```python
from build123d import *
from OCP.BRepFilletAPI import BRepFilletAPI_MakeChamfer

# Parameters (mm, degrees)
BOSS_EXTRUDE1_DEPTH     = 16.399996177
CUT_EXTRUDE1_DEPTH      = 32.345970628
CUT_EXTRUDE3_DEPTH      = 30.26106414
CUT_EXTRUDE3_DEPTH_BACK = 30.26106414
SKETCH4_R               = 1.7
BOSS_EXTRUDE2_START     = -4
BOSS_EXTRUDE2_DEPTH     = 4
FILLET1_R               = 12
CHAMFER1_SIZE           = 0.5
CHAMFER2_SIZE           = 0.5
CHAMFER2_SIZE2          = 1.366025404
MIRROR2_START           = 1.4
MIRROR2_DEPTH           = 9
CUT_EXTRUDE4_DEPTH      = 31.847364144
BOSS_EXTRUDE4_DEPTH     = 2.3
CHAMFER3_SIZE           = 2.3


# Read off the part's stored shape, not the designer's step: Mirror2
with BuildPart() as part:
    # Sketch1 → Boss-Extrude1 (new body)
    with BuildSketch(Plane.XY.offset(16.399996177)):
        with BuildLine():
            Line((7.2, 1.4), (22.5, 1.4))
            Line((22.5, 1.4), (22.5, 14.4))
            Line((22.5, 14.4), (7.2, 14.4))
            ThreePointArc((7.2, 14.4), (0.7, 7.9), (7.2, 1.4))
        make_face()
    extrude(amount=-BOSS_EXTRUDE1_DEPTH)

    # Sketch2 → Cut-Extrude1 (cut, through all)
    with BuildSketch(Plane(origin=(0, 0, 0), x_dir=(-1, 0, 0), z_dir=(0, 0, -1))):
        with BuildLine():
            Line((-22.5, 10.4), (-22.5, 5.4))
            Line((-22.5, 5.4), (-10.532688106, 5.4))
            ThreePointArc((-10.532688106, 5.4), (-2.9577807, 7.9), (-10.532688106, 10.4))
            Line((-10.532688106, 10.4), (-22.5, 10.4))
        make_face()
    extrude(amount=-CUT_EXTRUDE1_DEPTH, mode=Mode.SUBTRACT)

    # Sketch4 → Cut-Extrude3 (cut, two sides: drawn at the far end of the back side and taken through both)
    with BuildSketch(Plane.XZ.offset(-10.4).offset(-CUT_EXTRUDE3_DEPTH_BACK)):
        with Locations((19.72, 8.2)):
            Circle(SKETCH4_R)
    extrude(amount=CUT_EXTRUDE3_DEPTH + CUT_EXTRUDE3_DEPTH_BACK, mode=Mode.SUBTRACT)

    # Sketch5 → Boss-Extrude2 (add)
    with BuildSketch(Plane(origin=(0, 14.4, 0), x_dir=(1, 0, 0), z_dir=(0, 1, 0)).offset(BOSS_EXTRUDE2_START)):
        Polygon((22.5, 0), (22.5, -16.399996177), (27.234271104, -8.199998088), align=None)
    extrude(amount=BOSS_EXTRUDE2_DEPTH)

    # Fillet1
    fillet1_edges = [part.edges().sort_by_distance(p)[0] for p in [
        (27.234271104, 12.4, 8.199998088),
    ]]
    fillet(fillet1_edges, radius=FILLET1_R)

    # Chamfer1
    chamfer1_edges = [part.edges().sort_by_distance(p)[0] for p in [
        (2.9577807, 7.9, 16.399996177),
    ]]
    chamfer(chamfer1_edges, length=CHAMFER1_SIZE)

    # Chamfer2: one chamfer whose edges measure the first distance from different faces: ONE call of the kernel's chamfer builder (chamfer() names one face for all edges)
    chamfer2_edges_1 = [part.edges().sort_by_distance(p)[0] for p in [
        (22.5, 12.4, 16.399996177),
    ]]
    chamfer2_side_1 = [part.faces().sort_by_distance(p)[0] for p in [
        (23.135084744, 12.4, 15.299997133),
    ]]
    chamfer2_edges_2 = [part.edges().sort_by_distance(p)[0] for p in [
        (14.85, 1.4, 16.399996177),
        (0.7, 7.9, 16.399996177),
        (14.85, 14.4, 16.399996177),
        (16.818865224, 10.4, 16.399996177),
        (16.818865224, 5.4, 16.399996177),
    ]]
    chamfer2 = BRepFilletAPI_MakeChamfer(part.part.solid().wrapped)
    for e in chamfer2_edges_1:
        chamfer2.Add(CHAMFER2_SIZE, CHAMFER2_SIZE2, e.wrapped, chamfer2_side_1[0].wrapped)  # the first distance lies on this face
    for e in chamfer2_edges_2:
        chamfer2.Add(CHAMFER2_SIZE, e.wrapped)
    add(Compound.cast(chamfer2.Shape()), mode=Mode.REPLACE)

    # Mirror2 outline → Mirror2 (add)
    with BuildSketch(Plane(origin=(0, 0, 0), x_dir=(1, 0, 0), z_dir=(0, 1, 0)).offset(MIRROR2_START)):
        with BuildLine():
            ThreePointArc((23.770169489, -14.199998088), (25.377864643, -8.199998088), (23.770169489, -2.199998088))
            Line((23.770169489, -2.199998088), (22.5, 0))
            Line((22.5, 0), (22.5, -16.399996177))
            Line((22.5, -16.399996177), (23.770169489, -14.199998088))
        make_face()
    extrude(amount=MIRROR2_DEPTH)

    # Sketch7 → Cut-Extrude4 (cut, through all)
    with BuildSketch(Plane.ZY.offset(-22.5)):
        Polygon((0, 10.4), (0, 5.4), (15.899996177, 5.4), (16.399996177, 4.9), (16.399996177, 10.4), (15.899996177, 10.4), align=None)
    extrude(amount=-CUT_EXTRUDE4_DEPTH, mode=Mode.SUBTRACT)

    # Sketch9 → Boss-Extrude4 (add)
    with BuildSketch(Plane.XZ.offset(-1.4)):
        Polygon((16.891066023, 3.300146444), (22.548930666, 3.300144532), (25.377864643, 8.199998088), (22.548933977, 13.099853556), (16.891069334, 13.099855468), (14.062135357, 8.200001912), align=None)
        Polygon((21.32, 10.971281292), (18.12, 10.971281292), (16.52, 8.2), (18.12, 5.428718708), (21.32, 5.428718708), (22.92, 8.2), align=None, mode=Mode.SUBTRACT)
    extrude(amount=BOSS_EXTRUDE4_DEPTH)

    # Chamfer3
    # the kernel refuses this chamfer: 2.3 mm, written as the material it takes off along each edge
    with BuildSketch(Plane(origin=(19.591493499, -0.9, -1.822282904), x_dir=(0.023812122999065932, 0.9996219169112968, -0.013747946350707228), z_dir=(0.5000002926043912, 0, 0.8660252348491488))) as chamfer3_piece_1_section:
        Polygon((CHAMFER3_SIZE * 0.999621916911, CHAMFER3_SIZE * 0.0274958766106), (-CHAMFER3_SIZE * 0.0274958766106, CHAMFER3_SIZE * 0.999621916911), (0, 0), align=None)
    chamfer3_piece_1 = extrude(amount=17.487606388, mode=Mode.PRIVATE)
    chamfer3_piece_1 = split(chamfer3_piece_1, bisect_by=Plane(origin=(23.305279483, 1.4, 6.13003631), z_dir=(0, -1, 0)), keep=Keep.TOP, mode=Mode.PRIVATE)
    add(chamfer3_piece_1, mode=Mode.SUBTRACT)
    with BuildSketch(Plane(origin=(10.976195151, -0.9, 3.300148442), x_dir=(-9.290045060267903e-09, 0.9996219169112968, -0.027495876610584728), z_dir=(0.999999999999943, 0, -3.378704806423189e-07))) as chamfer3_piece_2_section:
        Polygon((CHAMFER3_SIZE * 0.999621916911, CHAMFER3_SIZE * 0.0274958766106), (-CHAMFER3_SIZE * 0.0274958766106, CHAMFER3_SIZE * 0.999621916911), (0, 0), align=None)
    chamfer3_piece_2 = extrude(amount=17.487606388, mode=Mode.PRIVATE)
    chamfer3_piece_2 = split(chamfer3_piece_2, bisect_by=Plane(origin=(19.719998601, 1.4, 4.060075043), z_dir=(0, -1, 0)), keep=Keep.TOP, mode=Mode.PRIVATE)
    add(chamfer3_piece_2, mode=Mode.SUBTRACT)
    with BuildSketch(Plane(origin=(11.104701651, -0.9, 13.322431346), x_dir=(-0.023812132289111273, 0.9996219169112968, -0.013747930259877354), z_dir=(0.49999970739555216, 0, -0.8660255727196295))) as chamfer3_piece_3_section:
        Polygon((CHAMFER3_SIZE * 0.999621916911, CHAMFER3_SIZE * 0.0274958766106), (-CHAMFER3_SIZE * 0.0274958766106, CHAMFER3_SIZE * 0.999621916911), (0, 0), align=None)
    chamfer3_piece_3 = extrude(amount=17.487606388, mode=Mode.PRIVATE)
    chamfer3_piece_3 = split(chamfer3_piece_3, bisect_by=Plane(origin=(16.134719118, 1.4, 6.130038733), z_dir=(0, -1, 0)), keep=Keep.TOP, mode=Mode.PRIVATE)
    add(chamfer3_piece_3, mode=Mode.SUBTRACT)
    with BuildSketch(Plane(origin=(19.848506501, -0.9, 18.222282904), x_dir=(-0.023812122999067282, 0.9996219169112966, 0.013747946350707963), z_dir=(-0.5000002926043904, 0, -0.8660252348491492))) as chamfer3_piece_4_section:
        Polygon((CHAMFER3_SIZE * 0.999621916911, CHAMFER3_SIZE * 0.0274958766106), (-CHAMFER3_SIZE * 0.0274958766106, CHAMFER3_SIZE * 0.999621916911), (0, 0), align=None)
    chamfer3_piece_4 = extrude(amount=17.487606388, mode=Mode.PRIVATE)
    chamfer3_piece_4 = split(chamfer3_piece_4, bisect_by=Plane(origin=(16.134720517, 1.4, 10.26996369), z_dir=(0, -1, 0)), keep=Keep.TOP, mode=Mode.PRIVATE)
    add(chamfer3_piece_4, mode=Mode.SUBTRACT)
    with BuildSketch(Plane(origin=(28.335298349, -0.9, 3.077568654), x_dir=(0.02381213228911159, 0.9996219169112966, 0.013747930259877545), z_dir=(-0.499999707395552, 0, 0.8660255727196297))) as chamfer3_piece_5_section:
        Polygon((CHAMFER3_SIZE * 0.999621916911, CHAMFER3_SIZE * 0.0274958766106), (-CHAMFER3_SIZE * 0.0274958766106, CHAMFER3_SIZE * 0.999621916911), (0, 0), align=None)
    chamfer3_piece_5 = extrude(amount=17.487606388, mode=Mode.PRIVATE)
    chamfer3_piece_5 = split(chamfer3_piece_5, bisect_by=Plane(origin=(23.305280882, 1.4, 10.269961267), z_dir=(0, -1, 0)), keep=Keep.TOP, mode=Mode.PRIVATE)
    add(chamfer3_piece_5, mode=Mode.SUBTRACT)
    with BuildSketch(Plane(origin=(28.463804849, -0.9, 13.099851558), x_dir=(9.290045031933457e-09, 0.9996219169112968, 0.027495876610584735), z_dir=(-0.9999999999999429, 0, 3.3787048064231847e-07))) as chamfer3_piece_6_section:
        Polygon((CHAMFER3_SIZE * 0.999621916911, CHAMFER3_SIZE * 0.0274958766106), (-CHAMFER3_SIZE * 0.0274958766106, CHAMFER3_SIZE * 0.999621916911), (0, 0), align=None)
    chamfer3_piece_6 = extrude(amount=17.487606388, mode=Mode.PRIVATE)
    chamfer3_piece_6 = split(chamfer3_piece_6, bisect_by=Plane(origin=(19.720001399, 1.4, 12.339924957), z_dir=(0, -1, 0)), keep=Keep.TOP, mode=Mode.PRIVATE)
    add(chamfer3_piece_6, mode=Mode.SUBTRACT)


solid = part.part
```
Geometry: final body of the model. Coordinates: model frame, mm. A direction names the side the tool comes from. Coordinates: 2 decimals unless noted, no trailing zeros. Loops run counter-clockwise (first coordinate to the right, second up) from the corner with the lowest first, then second, coordinate; pieces in that order, holes last. Notation, with made-up numbers: (87.25, 71.25) -> (109.25, 71.25) arc R29 ccw to (109.25, 96.25) -> close; hole circle Ø9 at (-18, 35). An arc over 180 degrees is marked (long way). Use a Markdown table: item, result. Add a question column.
(1) Access query for faces 4 (the flat face through (17.31, 0.35, 6.83)), 5 (the flat face through (23.25, 12.37, 15.1)), 6 (the flat face through (21.931, 12.373, 16.187)). Directions: +Z, -Z, +X, -X, +Y, -Y. A direction counts if a zero-diameter tool reaches every point of the face in a straight line with its end or side. Return the directions, or none.
(2) Line query: line 1 along Y through (x, z) = (21.5, 15.75); line 2 along X through (y, z) = (11.5, 8.25); line 3 along Y through (x, z) = (7, 5.25). Output: solid intervals per line, ascending.
(3) Mould query, pull axis Z, two halves, no side actions, for faces 1 (the flat face through (16.366, 0.351, 6.309)), 2 (the cylindrical face through (25.378, 12.428, 8.288)), 3 (the flat face through (20, 0, 10.971)). Classes: pulls with the +Z half, pulls with the -Z half, needs draft (parallel to the pull), parting line crosses it, or undercut.
(4) Section query A-A, the plane z = 8.5. Return loops of the section in (x, y), plus the area to 3 significant figures.
(5) Section query B-B, the plane y = 7.9. Return loops of the section in (x, z).
(6) Section query C-C, the plane z = 12.75. Return loops of the section in (x, y), plus the area to 3 significant figures.
(7) Section query D-D, the plane y = 4.5. State how many separate pieces and enclosed holes the cut face has, plus the area to 3 significant figures.
(8) Pin query (flat end, axial travel): pin 1 Ø4 at (y, z) = (9, 12.5) entering from +X; pin 2 Ø1.7 at (x, y) = (19.5, 0) entering from +Z; pin 3 Ø4 at (x, z) = (19.72, 8.2) entering from -Y; pin 4 Ø2.5 at (x, z) = (19.72, 8.2) entering from +Y. Return the tip coordinate at first contact, or that it passes through.
Answer:
| question | item | result |
|---|---|---|
| 1 | face 4 | -Y |
| 1 | face 5 | +Z, +X, +Y, -Y |
| 1 | face 6 | +Z, +X, +Y |
| 2 | line 1 | y = 1.4 to 5.4, 10.4 to 14.4 |
| 2 | line 2 | x = 1.79 to 4.99, 9.32 to 18.02, 21.42 to 25.38 |
| 2 | line 3 | y = 1.4 to 3.7, 12.1 to 14.4 |
| 3 | face 1 | pulls with the -Z half |
| 3 | face 2 | parting line crosses it |
| 3 | face 3 | undercut |
| 4 | outline | (7.2, 1.4) -> (14.24, 1.4) -> (16.69, -0.73) -> (16.69, 1.4) -> (18.05, 1.4) -> (18.05, 5.4) -> (10.53, 5.4) arc R4.2 cw (long way) to (10.53, 10.4) -> (18.05, 10.4) -> (18.05, 14.4) -> (7.2, 14.4) arc R6.5 ccw to start; (21.39, 1.4) -> (22.75, 1.4) -> (22.75, -0.73) -> (25.2, 1.4) -> (25.37, 1.4) -> (25.37, 5.4) -> (21.39, 5.4) -> close; (21.39, 10.4) -> (25.37, 10.4) -> (25.37, 14.4) -> (21.39, 14.4) -> close |
| 4 | area | 154 mm^2 |
| 5 | outline | (0.7, 0) -> (2.96, 0) -> (2.96, 15.9) -> (2.46, 16.4) -> (1.2, 16.4) -> (0.7, 15.9) -> close |
| 6 | outline | (7.2, 1.4) -> (16.69, 1.4) -> (17.09, 1.05) -> (22.35, 1.05) -> (22.75, 1.4) -> (24.48, 1.4) -> (24.48, 5.4) -> (10.53, 5.4) arc R4.2 cw (long way) to (10.53, 10.4) -> (24.48, 10.4) -> (24.48, 14.4) -> (7.2, 14.4) arc R6.5 ccw to start |
| 6 | area | 171 mm^2 |
| 7 | separate pieces | 2 |
| 7 | enclosed holes | 1 |
| 7 | area | 282 mm^2 |
| 8 | pin 1 | stops at x = 25.03 |
| 8 | pin 2 | stops at z = 12.55 |
| 8 | pin 3 | stops at y = 1.4 |
| 8 | pin 4 | passes through |
